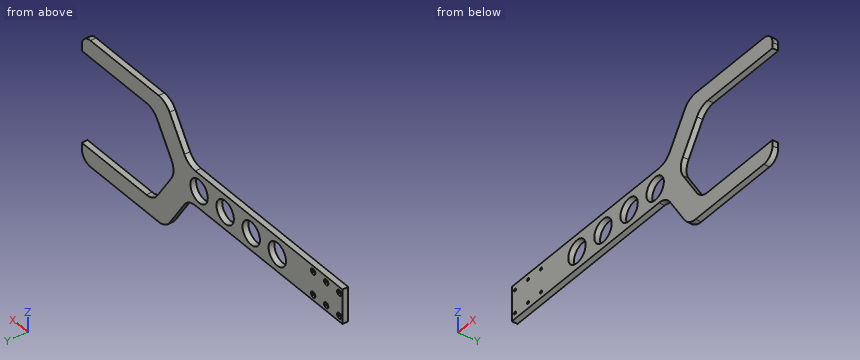
```python
from build123d import *

# Parameters (mm, degrees)
EXTRUDE_1_DEPTH     = 10
SKETCH_3_R          = 20
CUT_EXTRUDE_1_DEPTH = 611.081961707
SKETCH_4_R          = 5
CUT_EXTRUDE_2_DEPTH = 3
SKETCH_5_R          = 2.25
CUT_EXTRUDE_3_DEPTH = 611.040162612


with BuildPart() as part:
    # 스케치1 → 보스-돌출1 (new body)
    with BuildSketch(Plane(origin=(0, 0, 0), x_dir=(1, 0, 0), z_dir=(0, 1, 0))):
        with BuildLine():
            Line((363.866410807, 43.701562934), (397.902344915, 96.298437066))
            ThreePointArc((397.902344915, 96.298437066), (408.752779214, 106.352923101), (423.088868082, 110))
            Line((423.088868082, 110), (580, 110))
            ThreePointArc((580, 110), (594.142135624, 104.142135624), (600, 90))
            Line((600, 90), (600, 80))
            Line((600, 80), (451.32011236, 80))
            ThreePointArc((451.32011236, 80), (436.984023492, 76.352923101), (426.133589193, 66.298437066))
            Line((426.133589193, 66.298437066), (393.778116867, 16.298437066))
            ThreePointArc((393.778116867, 16.298437066), (388.964640033, 0), (393.778116867, -16.298437066))
            Line((393.778116867, -16.298437066), (426.133589193, -66.298437066))
            ThreePointArc((426.133589193, -66.298437066), (436.984023492, -76.352923101), (451.32011236, -80))
            Line((451.32011236, -80), (600, -80))
            Line((600, -80), (600, -90))
            ThreePointArc((600, -90), (594.142135624, -104.142135624), (580, -110))
            Line((580, -110), (423.088868082, -110))
            ThreePointArc((423.088868082, -110), (408.752779214, -106.352923101), (397.902344915, -96.298437066))
            Line((397.902344915, -96.298437066), (363.866410807, -43.701562934))
            ThreePointArc((363.866410807, -43.701562934), (353.015976508, -33.647076899), (338.67988764, -30))
            Line((338.67988764, -30), (0, -30))
            Line((0, -30), (0, 30))
            Line((0, 30), (338.67988764, 30))
            ThreePointArc((338.67988764, 30), (353.015976508, 33.647076899), (363.866410807, 43.701562934))
        make_face()
    extrude(amount=EXTRUDE_1_DEPTH)

    # 스케치3 → 컷-돌출1 (cut, through all)
    with BuildSketch(Plane(origin=(0, 10, 0), x_dir=(1, 0, 0), z_dir=(0, 1, 0))):
        with Locations(Location((150, 0, 0), (0, 0, 270))):
            Circle(SKETCH_3_R)
        with Locations(Location((210, 0, 0), (0, 0, 270))):
            Circle(SKETCH_3_R)
        with Locations(Location((270, 0, 0), (0, 0, 270))):
            Circle(SKETCH_3_R)
        with Locations(Location((330, 0, 0), (0, 0, 270))):
            Circle(SKETCH_3_R)
    extrude(amount=-CUT_EXTRUDE_1_DEPTH, mode=Mode.SUBTRACT)

    # 스케치4 → 컷-돌출2 (cut)
    with BuildSketch(Plane(origin=(0, 10, 0), x_dir=(1, 0, 0), z_dir=(0, 1, 0))):
        with Locations(Location((7.5, 20, 0), (0, 0, 270))):
            Circle(SKETCH_4_R)
        with Locations(Location((37.5, 20, 0), (0, 0, 270))):
            Circle(SKETCH_4_R)
        with Locations(Location((67.5, 20, 0), (0, 0, 270))):
            Circle(SKETCH_4_R)
        with Locations(Location((7.5, -20, 0), (0, 0, 270))):
            Circle(SKETCH_4_R)
        with Locations(Location((37.5, -20, 0), (0, 0, 270))):
            Circle(SKETCH_4_R)
        with Locations(Location((67.5, -20, 0), (0, 0, 270))):
            Circle(SKETCH_4_R)
    extrude(amount=-CUT_EXTRUDE_2_DEPTH, mode=Mode.SUBTRACT)

    # 스케치5 → 컷-돌출3 (cut, through all)
    with BuildSketch(Plane(origin=(0, 7, 0), x_dir=(1, 0, 0), z_dir=(0, 1, 0))):
        with Locations(Location((37.5, 20, 0), (0, 0, 270))):
            Circle(SKETCH_5_R)
        with Locations(Location((67.5, 20, 0), (0, 0, 270))):
            Circle(SKETCH_5_R)
        with Locations(Location((67.5, -20, 0), (0, 0, 270))):
            Circle(SKETCH_5_R)
        with Locations(Location((37.5, -20, 0), (0, 0, 270))):
            Circle(SKETCH_5_R)
        with Locations(Location((7.5, -20, 0), (0, 0, 270))):
            Circle(SKETCH_5_R)
        with Locations(Location((7.5, 20, 0), (0, 0, 270))):
            Circle(SKETCH_5_R)
    extrude(amount=-CUT_EXTRUDE_3_DEPTH, mode=Mode.SUBTRACT)


solid = part.part
```
CAD build for the part. Positions are in the model's coordinates, mm. Give positions to 0.01 mm unless a question says otherwise; leave off trailing zeros. Order: outer loops, then holes, each group sorted by start corner. A loop starts at its lowest first (then second) coordinate and runs counter-clockwise, first axis right, second up.
(1) Saw through at C-C, the plane y = 3.25. State how many separate pieces and enclosed holes the cut face has, then the cut area to 3 significant figures.
(2) Flat gauge pins, fed straight in: pin 1 (9 mm diameter, centred on x = 37.5, z = -20, fed in from +Y); pin 2 (5 mm diameter, centred on x = 222.5, y = 2.5, fed in from -Z); pin 3 (3 mm diameter, centred on x = 206.5, y = 6, fed in from +Z). Where does each tip first touch, or does it go through?
(3) Saw through at A-A, the plane z = 0. Give the cut face in (x, y), then the cut area to 3 significant figures.
(4) Saw through at B-B, the plane x = 270. Give the cut face in (y, z).
(5) Drill centre lines: L1, parallel to X at y = 3.25, z = 0; L2, parallel to X at y = 2.5, z = 12; L3, parallel to Z at x = 545.5, y = 4. Where is each one in solid material? Low to high.
(6) Saw through at D-D, the plane z = -50.5. Give the cut face in (x, y), then the cut area to 3 significant figures.
Results found:
1. separate pieces: 1
1. enclosed holes: 10
1. area: 35,400 mm2
2. pin 1: stops at y = 7
2. pin 2: stops at z = -30
2. pin 3: stops at z = 30
3. outline: (0, 0) - (130, 0) - (130, 10) - (0, 10) - close; (170, 0) - (190, 0) - (190, 10) - (170, 10) - close; (230, 0) - (250, 0) - (250, 10) - (230, 10) - close; (290, 0) - (310, 0) - (310, 10) - (290, 10) - close; (350, 0) - (388.96, 0) - (388.96, 10) - (350, 10) - close
3. area: 2,290 mm2
4. outline: (0, -30) - (10, -30) - (10, -20) - (0, -20) - close; (0, 20) - (10, 20) - (10, 30) - (0, 30) - close
5. L1: x = 0 to 130, 170 to 190, 230 to 250, 290 to 310, 350 to 388.96
5. L2: x = 0 to 134, 166 to 194, 226 to 254, 286 to 314, 346 to 391.47
5. L3: z = -110 to -80, 80 to 110
6. outline: (368.27, 0) - (415.91, 0) - (415.91, 10) - (368.27, 10) - close
6. area: 476 mm2
